Here's how the part is built. I have some questions about the finished solid (model axes, mm). A direction names the side the tool comes from. Coordinates: 2 decimals unless noted, no trailing zeros. Write each loop counter-clockwise with the first axis right and the second up, starting at its lowest first coordinate (ties: lowest second). Pieces come first, ordered by that corner, then holes. Notation, with made-up numbers: (8, -8.5) - (48, -8.5) arc R26 ccw to (48, 27.5) - close; hole circle Ø2 at (47, -16.75). An arc over 180 degrees is marked (long way). Answer in a Markdown table with one row per item. Add a question column.
Item 1: I'm going to push flat-ended pins straight in: pin 1 (1 mm diameter, centred on x = -3.5, y = 41, fed in from -Z); pin 2 (3 mm diameter, centred on y = 18, z = 0.5, fed in from +X); pin 3 (2 mm diameter, centred on y = 12, z = -9.5, fed in from +X); pin 4 (1 mm diameter, centred on x = 10, y = 49, fed in from -Z). Where does each tip first touch, or does it pass through?
Item 2: Imagine slicing it at D-D (y = 40). Please give me the cut outline in (x, z), plus the area to 3 significant figures.
Item 3: Imagine slicing it at B-B (y = 6.5). Please give me the cut outline in (x, z), plus the area to 3 significant figures.
Item 4: Which directions (+Z, -Z, +X, -X, +Y, -Y) give clear straight access to the entire face, cutting with the end or side of a thin tool? Please do faces 4 (the face through (0, 56, 0)), 5 (the face through (6.466, 22.888, -2.681)).
Item 5: We'd pull the mould along X, two halves only. Please class faces 1 (the face through (-1, 0, 12.3)), 2 (the face through (2.981, 24.65, 13.423)), 3 (the face through (5.2, 15, -5.2)): +X half, -X half, draft (parallel to the pull), parting line (faces both ways), or undercut.
Item 6: Imagine slicing it at C-C (z = 0). Please give me the cut outline in (x, y), plus the area to 3 significant figures.
Item 7: Imagine slicing it at A-A (x = 0). Please give me the cut outline in (y, z), plus the area to 3 significant figures.
Item 8: If I drill on probe 1 along Z at (x, y) = (0.5, 14); probe 2 along Z at (x, y) = (0, 23); probe 3 along Y at (x, z) = (7, -2.75), over which ranges is the centre line in solid material (lowest first)? Write a range as from..to.
Autodesk Inventor part; units mm, degrees
ref_plane "YZ Plane" through (0, 0, 0) normal (1, 0, 0) x (0, 1, 0)
ref_plane "XZ Plane" through (0, 0, 0) normal (0, 1, 0) x (-1, 0, 0)
ref_plane "XY Plane" through (0, 0, 0) normal (0, 0, 1) x (1, 0, 0)
sketch "Sketch1" plane through (0, 0, 0) normal (0, 1, 0) x (-1, 0, 0)
  circle A0 centre (0, 0) radius 13.75
  dimension "d0" = 27.5
extrude "Extrusion1" add sketch "Sketch1" along normal blind 56
fillet "Fillet1" radius 6 1 edges at (13.75, 56, 0)
sketch "Sketch2" plane through (0, 0, 0) normal (0, -1, 0) x (1, 0, 0)
  circle A0 centre (0, 0) radius 12
  dimension "d4" = 24
extrude "Extrusion2" cut sketch "Sketch2" against normal blind 15
sketch "Sketch3" plane through (0, 15, 0) normal (0, -1, 0) x (1, 0, 0)
  circle A0 centre (0, 0) radius 7
  dimension "d7" = 14
extrude "Extrusion3" cut sketch "Sketch3" against normal blind 16
properties part number "E14 socket"
Here are the results:
| question | item | result |
|---|---|---|
| 1 | pin 1 | stops at z = -13.42 |
| 1 | pin 2 | stops at x = 13.75 |
| 1 | pin 3 | stops at x = 10.81 |
| 1 | pin 4 | stops at z = -9.94 |
| 2 | outline | circle Ø27.5 at (0, 0) |
| 2 | area | 594 mm2 |
| 3 | outline | circle Ø27.5 at (0, 0); hole circle Ø24 at (0, 0) |
| 3 | area | 142 mm2 |
| 4 | face 4 | +Z, -Z, +X, -X, +Y |
| 4 | face 5 | -Y |
| 5 | face 1 | draft |
| 5 | face 2 | parting line |
| 5 | face 3 | undercut |
| 6 | outline | (-13.75, 0) - (-12, 0) - (-12, 15) - (-7, 15) - (-7, 31) - (7, 31) - (7, 15) - (12, 15) - (12, 0) - (13.75, 0) - (13.75, 50) arc R6 ccw to (7.75, 56) - (-7.75, 56) arc R6 ccw to (-13.75, 50) - close |
| 6 | area | 941 mm2 |
| 7 | outline | (0, -13.75) - (50, -13.75) arc R6 ccw to (56, -7.75) - (56, 7.75) arc R6 ccw to (50, 13.75) - (0, 13.75) - (0, 12) - (15, 12) - (15, 7) - (31, 7) - (31, -7) - (15, -7) - (15, -12) - (0, -12) - close |
| 7 | area | 941 mm2 |
| 8 | probe 1 | z = -13.74..-11.99, 11.99..13.74 |
| 8 | probe 2 | z = -13.75..-7, 7..13.75 |
| 8 | probe 3 | y = 15..56 |
